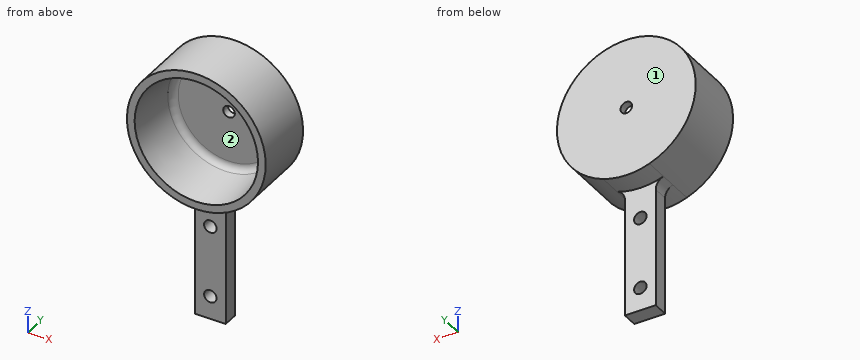
from build123d import *
from build123d import SkipClean  # not in build123d's __all__

# Parameters (mm, degrees)
F0_R     = 2.5781
F0_R_2   = 2.38125
F2_DEPTH = 25.4
F4_R     = 2.5781
F5_DEPTH = 9.525
F6_R     = 2.5781
F7_DEPTH = 9.525


with BuildPart() as f2:
    # F0 (on Front) → F2 (new body)
    with BuildSketch(Plane.XZ):
        with BuildLine():
            ThreePointArc((6.35, -31.4308964237), (7.2239350333, -28.6812657667), (9.525, -26.9407683632))
            ThreePointArc((9.525, -26.9407683632), (0, 28.575), (-9.525, -26.9407683632))
            ThreePointArc((-9.525, -26.9407683632), (-7.2239350333, -28.6812657667), (-6.35, -31.4308964237))
            Line((-6.35, -31.4308964237), (-6.35, -80.264))
            Line((-6.35, -80.264), (6.35, -80.264))
            Line((6.35, -80.264), (6.35, -31.4308964237))
        make_face()
        with Locations((0, -70.739)):
            Circle(F0_R, mode=Mode.SUBTRACT)
        with Locations((0, -41.275)):
            Circle(F0_R, mode=Mode.SUBTRACT)
        Circle(F0_R_2, mode=Mode.SUBTRACT)
    extrude(amount=-F2_DEPTH)

    # F1 (on Right) → F3 (revolve, cut)
    with BuildSketch(Plane.YZ):
        with BuildLine():
            Line((19.6890045478, 23.677435306), (0, 25.4))
            Line((0, 25.4), (0, 0))
            Line((0, 0), (22.225, 0))
            Line((22.225, 0), (22.225, 20.9098819103))
            ThreePointArc((22.225, 20.9098819103), (21.4951236013, 22.7867559559), (19.6890045478, 23.677435306))
        make_face()
    revolve(axis=Axis((0, 12.7, 0), (0, 1, 0)), mode=Mode.SUBTRACT)

    # F4 (on face) → F5 (cut)
    with BuildSketch(Plane.XZ):
        with BuildLine():
            ThreePointArc((9.525, -26.9407683632), (0, -28.575), (-9.525, -26.9407683632))
            ThreePointArc((-9.525, -26.9407683632), (-7.2239350333, -28.6812657667), (-6.35, -31.4308964237))
            Line((-6.35, -31.4308964237), (-6.35, -80.264))
            Line((-6.35, -80.264), (6.35, -80.264))
            Line((6.35, -80.264), (6.35, -31.4308964237))
            ThreePointArc((6.35, -31.4308964237), (7.2239350333, -28.6812657667), (9.525, -26.9407683632))
        make_face()
        with Locations((0, -70.739)):
            Circle(F4_R, mode=Mode.SUBTRACT)
        with Locations((0, -41.275)):
            Circle(F4_R, mode=Mode.SUBTRACT)
    with SkipClean():  # cleaning this boolean's faces spoils the solid; the shape is the same uncleaned
        extrude(amount=-F5_DEPTH, mode=Mode.SUBTRACT)

    # F6 (on face) → F7 (cut)
    with BuildSketch(Plane(origin=(0, 25.4, 0), x_dir=(-1, 0, 0), z_dir=(0, 1, 0))):
        with BuildLine():
            ThreePointArc((9.525, -26.9407683632), (0, -28.575), (-9.525, -26.9407683632))
            ThreePointArc((-9.525, -26.9407683632), (-7.2239350333, -28.6812657667), (-6.35, -31.4308964237))
            Line((-6.35, -31.4308964237), (-6.35, -80.264))
            Line((-6.35, -80.264), (6.35, -80.264))
            Line((6.35, -80.264), (6.35, -31.4308964237))
            ThreePointArc((6.35, -31.4308964237), (7.2239350333, -28.6812657667), (9.525, -26.9407683632))
        make_face()
        with Locations((0, -70.739)):
            Circle(F6_R, mode=Mode.SUBTRACT)
        with Locations((0, -41.275)):
            Circle(F6_R, mode=Mode.SUBTRACT)
    extrude(amount=-F7_DEPTH, mode=Mode.SUBTRACT)


solid = f2.part
Can you work these out from the model? Positions are in its coordinate system, mm. Face numbers are marked on the shaded views. Coordinates: 2 decimals unless noted, no trailing zeros. Order: outer loops, then holes, each group sorted by start corner. A loop starts at its lowest first (then second) coordinate and runs counter-clockwise, first axis right, second up. Notation, with made-up numbers: (41, 45) - (50, 45) arc R9 cw to (50, 61) - close; hole circle Ø3 at (87.25, 85.25). An arc over 180 degrees is marked (long way). Answer as a JSON object with one key per item and string values. Group by question number.
Q1. Imagine slicing it at D-D (z = -60). Please give me the cut outline in (x, y) (3 decimals).
Q2. Will these pins go through, and if not, where does the flat tip stop? P1, Ø10, axis at x = -4.5, y = 7.5, coming from the -Z side; P2, Ø10, axis at y = 22.5, z = -40, coming from the -X side; P3, Ø1, axis at y = 14, z = -2, coming from the +X side; P4, Ø6, axis at x = 0, z = -70.739, coming from the +Y side (3 decimals).
Q3. Imagine slicing it at C-C (y = 7.5). Please give me the cut outline in (x, z) (3 decimals), and give its area (3 significant figures).
Q4. We'd pull the mould along X, two halves only. Please class the marked faces 1 and 2: +X half, -X half, draft (parallel to the pull), parting line (faces both ways), or undercut.
Q5. Imagine slicing it at B-B (x = 0). Please give me the cut outline in (y, z) (3 decimals).
Q6. I need wall thicknesses on line 1 (Z direction, x = 0, y = 24.45) (3 decimals); line 2 (Z direction, x = -2, y = 11.5); line 3 (Y direction, x = 15.5, z = 13) (3 decimals). Which ranges of each line are inside material? Lowest first, please. Write a range as from..to.
Q7. Imagine slicing it at A-A (z = 0). Please give me the cut outline in (x, y) (3 decimals).
Determined:
{
 "1": {"outline": "(-6.35, 9.525) - (6.35, 9.525) - (6.35, 15.875) - (-6.35, 15.875) - close"},
 "2": {"P1": "stops at z = -80.26", "P2": "passes through", "P3": "stops at x = 28.54", "P4": "stops at y = 15.875"},
 "3": {"outline": "circle Ø57.15 at (0, 0); hole circle Ø49.488 at (0, 0)", "area": "642 mm2"},
 "4": {"face 1": "draft", "face 2": "undercut"},
 "5": {"outline": "(0, -28.575) - (9.525, -28.575) - (9.525, -38.697) - (15.875, -38.697) - (15.875, -28.575) - (25.4, -28.575) - (25.4, -2.381) - (22.225, -2.381) - (22.225, -20.91) arc R2.778 cw to (19.689, -23.677) - (0, -25.4) - close; (0, 25.4) - (19.689, 23.677) arc R2.778 cw to (22.225, 20.91) - (22.225, 2.381) - (25.4, 2.381) - (25.4, 28.575) - (0, 28.575) - close; (9.525, -80.264) - (15.875, -80.264) - (15.875, -73.317) - (9.525, -73.317) - close; (9.525, -68.161) - (15.875, -68.161) - (15.875, -43.853) - (9.525, -43.853) - close"},
 "6": {"line 1": "z = -28.575..-2.381, 2.381..28.575", "line 2": "z = -80.26..-72.37, -69.11..-42.9, -39.65..-24.31, 24.31..28.5", "line 3": "y = 22.225..25.4"},
 "7": {"outline": "(-28.575, 0) - (-25.4, 0) - (-23.677, 19.689) arc R2.778 cw to (-20.91, 22.225) - (-2.381, 22.225) - (-2.381, 25.4) - (-28.575, 25.4) - close; (2.381, 22.225) - (20.91, 22.225) arc R2.778 cw to (23.677, 19.689) - (25.4, 0) - (28.575, 0) - (28.575, 25.4) - (2.381, 25.4) - close"}
}
